Geometry check sheet. Reference: the model listing, model coordinates, mm. A direction names the side the tool comes from. Coordinates: 2 decimals unless noted, no trailing zeros. Loops run counter-clockwise (first coordinate to the right, second up) from the corner with the lowest first, then second, coordinate; pieces in that order, holes last. Notation, with made-up numbers: (78.5, 78) -> (86.5, 78) arc R23 cw to (86.5, 102) -> close; hole circle Ø11 at (-11.75, 17). An arc over 180 degrees is marked (long way). Answer as a JSON object with one key per item and string values.
from build123d import *

# Parameters (mm, degrees)
SKETCH1_W           = 150
SKETCH1_H           = 35
SKETCH1_W_2         = 38
SKETCH1_H_2         = 30
SKETCH1_W_3         = 25
SKETCH1_H_3         = 15
SKETCH1_W_4         = 15
BOSS_EXTRUDE1_DEPTH = 10
SKETCH2_W           = 25
SKETCH2_H           = 15
SKETCH2_W_2         = 38
SKETCH2_H_2         = 30
SKETCH2_W_3         = 15
BOSS_EXTRUDE2_DEPTH = 2
SKETCH3_W           = 19
SKETCH3_H           = 2.5
CUT_EXTRUDE3_DEPTH  = 8
FILLET1_START       = -75
FILLET1_DEPTH       = 150
FILLET1_START_2     = -18
FILLET1_2_DEPTH     = 36
FILLET2_R           = 5


with BuildPart() as part:
    # Sketch1 → Boss-Extrude1 (new body)
    with BuildSketch(Plane(origin=(0, 0, 0), x_dir=(1, 0, 0), z_dir=(0, 1, 0))):
        Rectangle(SKETCH1_W, SKETCH1_H)
        Rectangle(SKETCH1_W_2, SKETCH1_H_2, mode=Mode.SUBTRACT)
        with Locations((-37.5, 0)):
            Rectangle(SKETCH1_W_3, SKETCH1_H_3, mode=Mode.SUBTRACT)
        with Locations((37.5, 0)):
            Rectangle(SKETCH1_W_4, SKETCH1_H_3, mode=Mode.SUBTRACT)
    extrude(amount=BOSS_EXTRUDE1_DEPTH)

    # Sketch2 → Boss-Extrude2 (add)
    with BuildSketch(Plane.XZ):
        with Locations((-37.5, 0)):
            Rectangle(SKETCH2_W, SKETCH2_H)
        Rectangle(SKETCH2_W_2, SKETCH2_H_2)
        with Locations((37.5, 0)):
            Rectangle(SKETCH2_W_3, SKETCH2_H)
    extrude(amount=-BOSS_EXTRUDE2_DEPTH)

    # Sketch3 → Cut-Extrude3 (cut)
    with BuildSketch(Plane(origin=(0, 2, 0), x_dir=(1, 0, 0), z_dir=(0, 1, 0))):
        with Locations((-9.5, 16.25)):
            Rectangle(SKETCH3_W, SKETCH3_H)
    extrude(amount=CUT_EXTRUDE3_DEPTH, mode=Mode.SUBTRACT)

    # Fillet1: read off the stored shape, not the designer's step
    # Fillet1 outline → Fillet1 (cut)
    with BuildSketch(Plane.YZ.offset(FILLET1_START)):
        with BuildLine():
            Line((10, -17.5), (10, -15))
            ThreePointArc((10, -15), (9.267766953, -16.767766953), (7.5, -17.5))
            Line((7.5, -17.5), (10, -17.5))
        make_face()
        with BuildLine():
            ThreePointArc((7.5, 17.5), (9.267766953, 16.767766953), (10, 15))
            Line((10, 15), (10, 17.5))
            Line((10, 17.5), (7.5, 17.5))
        make_face()
    extrude(amount=FILLET1_DEPTH, mode=Mode.SUBTRACT)

    # Fillet1 2 outline → Fillet1 2 (cut)
    with BuildSketch(Plane.XY.offset(FILLET1_START_2)):
        with BuildLine():
            Line((75, 10), (72.5, 10))
            ThreePointArc((72.5, 10), (74.267766953, 9.267766953), (75, 7.5))
            Line((75, 7.5), (75, 10))
        make_face()
        with BuildLine():
            ThreePointArc((-75, 7.5), (-74.267766953, 9.267766953), (-72.5, 10))
            Line((-72.5, 10), (-75, 10))
            Line((-75, 10), (-75, 7.5))
        make_face()
    extrude(amount=FILLET1_2_DEPTH, mode=Mode.SUBTRACT)

    # Fillet2
    # the kernel refuses this fillet: 5 mm, written as the material it takes off along each edge
    with BuildSketch(Plane(origin=(70, 10, -12.5), x_dir=(1, 0, 0), z_dir=(0, 0, 1))) as fillet2_piece_1:
        with BuildLine():
            CenterArc((2.5, -2.5), 2.5, 0, 90)
            Line((5, -2.5), (5, 0))
            Line((5, 0), (2.5, 0))
        make_face()
    revolve(axis=Axis((70, 10, -12.5), (0, 1, 0)), revolution_arc=90, mode=Mode.SUBTRACT)
    with BuildSketch(Plane(origin=(70, 10, 12.5), x_dir=(0, 0, 1), z_dir=(-1, 0, 0))) as fillet2_piece_2:
        with BuildLine():
            CenterArc((2.5, -2.5), 2.5, 0, 90)
            Line((5, -2.5), (5, 0))
            Line((5, 0), (2.5, 0))
        make_face()
    revolve(axis=Axis((70, 10, 12.5), (0, 1, 0)), revolution_arc=90, mode=Mode.SUBTRACT)
    with BuildSketch(Plane(origin=(-70, 10, -12.5), x_dir=(0, 0, -1), z_dir=(1, 0, 0))) as fillet2_piece_3:
        with BuildLine():
            CenterArc((2.5, -2.5), 2.5, 0, 90)
            Line((5, -2.5), (5, 0))
            Line((5, 0), (2.5, 0))
        make_face()
    revolve(axis=Axis((-70, 10, -12.5), (0, 1, 0)), revolution_arc=90, mode=Mode.SUBTRACT)
    with BuildSketch(Plane(origin=(-70, 10, 12.5), x_dir=(-1, 0, 0), z_dir=(0, 0, -1))) as fillet2_piece_4:
        with BuildLine():
            CenterArc((2.5, -2.5), 2.5, 0, 90)
            Line((5, -2.5), (5, 0))
            Line((5, 0), (2.5, 0))
        make_face()
    revolve(axis=Axis((-70, 10, 12.5), (0, 1, 0)), revolution_arc=90, mode=Mode.SUBTRACT)
    with BuildSketch(Plane(origin=(-75, -12.5, 17.5), x_dir=(1, 0, 0), z_dir=(0, 1, 0)), Plane(origin=(-75, -12.5, -17.5), x_dir=(0, 0, 1), z_dir=(0, 1, 0))) as fillet2_piece_5:
        with BuildLine():
            CenterArc((FILLET2_R, FILLET2_R), FILLET2_R, 180, 90)
            Line((0, FILLET2_R), (0, 0))
            Line((0, 0), (FILLET2_R, 0))
        make_face()
    extrude(amount=22.5, mode=Mode.SUBTRACT)
    with BuildSketch(Plane(origin=(75, -12.5, -17.5), x_dir=(0, 0, 1), z_dir=(0, 1, 0)), Plane(origin=(75, -12.5, 17.5), x_dir=(-1, 0, 0), z_dir=(0, 1, 0))) as fillet2_piece_6:
        with BuildLine():
            CenterArc((FILLET2_R, -FILLET2_R), FILLET2_R, 90, 90)
            Line((0, -FILLET2_R), (0, 0))
            Line((0, 0), (FILLET2_R, 0))
        make_face()
    extrude(amount=22.5, mode=Mode.SUBTRACT)


solid = part.part
1. Section check C-C, the plane z = -10. Record the boundary of the cut face in (x, y), then the cut area to 3 significant figures.
Evaluation:
{"outline": "(-75, 0) -> (75, 0) -> (75, 7.5) arc R2.5 ccw to (72.5, 10) -> (19, 10) -> (19, 2) -> (-19, 2) -> (-19, 10) -> (-72.5, 10) arc R2.5 ccw to (-75, 7.5) -> close", "area": "1,190 mm^2"}
2. Thickness scan on probe 1 along X at (y, z) = (2.5, -4.5); probe 2 along X at (y, z) = (2.5, -10.5); probe 3 along Z at (x, y) = (41.5, 3.25). Record the ranges inside material, lowest first. Write a range as from..to.
Evaluation:
{"probe 1": "x = -75..-50, -25..-19, 19..30, 45..75", "probe 2": "x = -75..-19, 19..75", "probe 3": "z = -17.5..-7.5, 7.5..17.5"}
3. Tool access check on faces 4 (the face through (-1, 1, -17.5)), 5 (the face through (37, 6, -7.5)), 6 (the face through (-19, 6, -1)). Record the directions out of +Z, -Z, +X, -X, +Y, -Y that give a thin tool (end or side, any length) a straight path to the whole face; none if there is none.
Evaluation:
{"face 4": "-Z, +X, -X, +Y, -Y", "face 5": "+Y", "face 6": "-Z, +Y"}
4. Section check A-A, the plane x = 34. Record the boundary of the cut face in (y, z), then the cut area to 3 significant figures.
Evaluation:
{"outline": "(0, -17.5) -> (7.5, -17.5) arc R2.5 ccw to (10, -15) -> (10, -7.5) -> (2, -7.5) -> (2, 7.5) -> (10, 7.5) -> (10, 15) arc R2.5 ccw to (7.5, 17.5) -> (0, 17.5) -> close", "area": "227 mm^2"}
5. Section check B-B, the plane y = 3.75. Record the boundary of the cut face in (x, z), then the cut area to 3 significant figures.
Evaluation:
{"outline": "(-75, -12.5) arc R5 ccw to (-70, -17.5) -> (-19, -17.5) -> (-19, 15) -> (19, 15) -> (19, -15) -> (0, -15) -> (0, -17.5) -> (70, -17.5) arc R5 ccw to (75, -12.5) -> (75, 12.5) arc R5 ccw to (70, 17.5) -> (-70, 17.5) arc R5 ccw to (-75, 12.5) -> close; hole (-50, -7.5) -> (-25, -7.5) -> (-25, 7.5) -> (-50, 7.5) -> close; hole (30, -7.5) -> (45, -7.5) -> (45, 7.5) -> (30, 7.5) -> close", "area": "3,440 mm^2"}
6. Depth check by flat-ended pin: P1, Ø10, axis at x = 4, z = 5, coming from the +Y side; P2, Ø1.5, axis at y = 9, z = 2, coming from the -X side. Enter the tip coordinate at first touch or a pass-through.
Evaluation:
{"P1": "stops at y = 2", "P2": "stops at x = -74.88"}
7. Mould release check, pull along X, two halves, no side actions. Record for faces 1 (the face through (-45, 9, -17)), 2 (the face through (37, 2, 0)), 3 (the face through (-73.5, 3.7, -16.07)): released by +X, released by -X, zero draft, split by the parting line, or undercut.
Evaluation:
{"face 1": "zero draft", "face 2": "undercut", "face 3": "released by -X"}
8. Section check D-D, the plane z = 2. Record the boundary of the cut face in (x, y), then the cut area to 3 significant figures.
Evaluation:
{"outline": "(-75, 0) -> (75, 0) -> (75, 7.5) arc R2.5 ccw to (72.5, 10) -> (45, 10) -> (45, 2) -> (30, 2) -> (30, 10) -> (19, 10) -> (19, 2) -> (-19, 2) -> (-19, 10) -> (-25, 10) -> (-25, 2) -> (-50, 2) -> (-50, 10) -> (-72.5, 10) arc R2.5 ccw to (-75, 7.5) -> close", "area": "873 mm^2"}
